Can you work these out from the model? Positions are in its coordinate system, mm. A direction names the side the tool comes from. Round coordinates to 2 decimals unless told otherwise and drop trailing zeros. Order: outer loops, then holes, each group sorted by start corner. A loop starts at its lowest first (then second) coordinate and runs counter-clockwise, first axis right, second up. Notation, with made-up numbers: M -36,-37 L -20,-37 A7 cw -20,-26 Z; hole C 1,10.25 d6. An arc over 180 degrees is marked long. One line per question, with ' | ' between items.
```python
from build123d import *

# Parameters (mm, degrees)
F1_DEPTH = 12.7
F3_DEPTH = 25.4
F4_DEPTH = 12.7
F5_R     = 7.3111886468
F6_DEPTH = 28.448


with BuildPart() as f1:
    # F0 (on Front) → F1 (new body)
    with BuildSketch(Plane.XZ):
        Polygon((-65.437734127, 0), (0, 0), (-32.6272174716, 66.4458796382), (-65.437734127, 66.4458796382), align=None)
    extrude(amount=F1_DEPTH)

    # F2 (on face) → F3 (join)
    with BuildSketch(Plane.XZ.offset(12.7)):
        Polygon((-59.5721639693, 0), (-13.0142271519, 0), (-33.360414207, 45.3664921224), (-59.5721639693, 45.3664921224), align=None)
    extrude(amount=F3_DEPTH)

    # F4 (add): a face of the model
    f4_faces = [f1.faces().sort_by_distance(p)[0] for p in [
        (-40.9056812293, -38.1, 20.569190108),
    ]]
    extrude(f4_faces, amount=F4_DEPTH)

    # F5 (on face) → F6 (cut)
    with BuildSketch(Plane(origin=(-10.8349077523, 0, -4.8592926087), x_dir=(0, 1, 0), z_dir=(0.9124381131, 0, 0.4092147234))):
        with Locations((-31.3933752477, 30.4919779301)):
            Circle(F5_R)
    extrude(amount=-F6_DEPTH, mode=Mode.SUBTRACT)


solid = f1.part
```
(1) If we section it at A-A on x = -53.5: Please give me the cut outline in (y, z).
Final values:
outline: M -50.8,0 L 0,0 L 0,66.45 L -12.7,66.45 L -12.7,45.37 L -50.8,45.37 Z
(2) If we section it at D-D on x = -60.5: Please give me the cut outline in (y, z), plus the area to 3 significant figures.
Final values:
outline: M -12.7,0 L 0,0 L 0,66.45 L -12.7,66.45 Z | area: 844 mm^2
(3) If we section it at C-C on z = 40.5: Please give me the cut outline in (x, y), plus the area to 3 significant figures.
Final values:
outline: M -65.44,-12.7 L -59.57,-12.7 L -59.57,-50.8 L -31.18,-50.8 L -31.18,-12.7 L -19.89,-12.7 L -19.89,0 L -65.44,0 Z | area: 1,660 mm^2
(4) Please list where these lines run through material, in increasing order: probe 1 along Z at (x, y) = (-55, -28); probe 2 along Y at (x, z) = (-26, 33); probe 3 along Y at (x, z) = (-33, 17). Write a range as [from, to].
Final values:
probe 1: [0, 45.37] | probe 2: [-12.7, 0] | probe 3: [-50.8, -38.55], [-24.23, 0]
(5) Thinking about a two-plate mould opening in Y: for faces 5 (the flat face through (-16.085, -6.261, 32.758)), 6 (the flat face through (-42, -50.8, 23)), 7 (the cylindrical face through (-36.2, -38.7, 17.5)), 8 (the flat face through (-49.31, -31.5, 11.41)), which applies, released by +Y, released by -Y, zero draft, split by the parting line, or undercut?
Final values:
face 5: zero draft | face 6: released by -Y | face 7: undercut | face 8: undercut
(6) On a 3-axis mill with a long thin cutter (end or side, diameter ignored), from which of +Z, -Z, +X, -X, +Y, -Y can I reach the whole of each face in a straight line? I mean faces 1 (the flat face through (-20.78, -35.72, 17.32)), 2 (the flat face through (-46, -31, 45.366)), 3 (the flat face through (-49, -6, 66.446)), 4 (the flat face through (-59.572, -31, 23)). Say none if no direction works.
Final values:
face 1: +Z, +X, -Y | face 2: +Z, +X, -X, -Y | face 3: +Z, +X, -X, +Y, -Y | face 4: +Z, -Z, -X, -Y
(7) If we section it at B-B on y = -43: Please give me the cut outline in (x, z).
Final values:
outline: M -59.57,0 L -13.01,0 L -33.36,45.37 L -59.57,45.37 Z
(8) Will these pins go through, and if not, where does the flat tip stop? pin 1 Ø19 at (y, z) = (-36, 23.5) entering from -X; pin 2 Ø5 at (y, z) = (-41, 42) entering from +X; pin 3 Ø4 at (y, z) = (-23, 35.5) entering from +X.
Final values:
pin 1: x = -59.57 | pin 2: x = -30.73 | pin 3: x = -28.04
